Geometry check sheet. Reference: the model listing, model coordinates, mm. Give positions to 0.01 mm unless a question says otherwise; leave off trailing zeros. Write each loop counter-clockwise with the first axis right and the second up, starting at its lowest first coordinate (ties: lowest second). Pieces come first, ordered by that corner, then holes. Notation, with made-up numbers: M 34,-6.5 L 72,-6.5 A25 ccw 72,9.5 Z; hole C 58.25,39.25 d5. An arc over 180 degrees is marked long. Write each question's results on one line, items separated by ' | '.
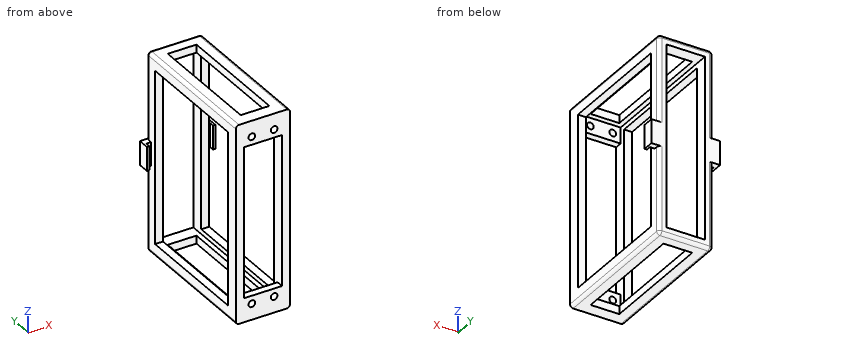
Autodesk Inventor part; units mm, degrees
ref_plane "YZ Plane" through (0, 0, 0) normal (1, 0, 0) x (0, 1, 0)
ref_plane "XZ Plane" through (0, 0, 0) normal (0, 1, 0) x (-1, 0, 0)
ref_plane "XY Plane" through (0, 0, 0) normal (0, 0, 1) x (1, 0, 0)
sketch "Sketch1" plane through (0, 0, 0) normal (0, 1, 0) x (-1, 0, 0)
  point P0 (0, 0)
sketch "Sketch2" plane through (0, 0, 0) normal (0, 1, 0) x (-1, 0, 0)
  line L0 (34.7144, 60.4703) -> (0.7144, 60.4703)
  line L1 (0.7144, 60.4703) -> (0.7144, -63.8297)
  line L2 (0.7144, -63.8297) -> (34.7144, -63.8297)
  line L3 (34.7144, -63.8297) -> (34.7144, 60.4703)
  point P0 (0, 0)
  dimension "d0" = 124.3
  dimension "d1" = 34
extrude "Extrusion1" add sketch "Sketch2" along normal blind 90
sketch "Sketch3" plane through (0, 90, 0) normal (0, 1, 0) x (1, 0, 0)
  line L0 (-34.7144, -60.4703) -> (-0.7144, -60.4703) construction
  line L1 (-0.7144, -60.4703) -> (-0.7144, 63.8297) construction
  line L2 (-0.7144, 63.8297) -> (-34.7144, 63.8297) construction
  line L3 (-34.7144, 63.8297) -> (-34.7144, -60.4703) construction
  line L4 (-29.7144, 58.8297) -> (-5.7144, 58.8297)
  line L5 (-5.7144, 58.8297) -> (-5.7144, -55.4703)
  line L6 (-5.7144, -55.4703) -> (-29.7144, -55.4703)
  line L7 (-29.7144, -55.4703) -> (-29.7144, 58.8297)
  point P0 (0, 0)
  dimension "d4" = 114.3
  dimension "d5" = 24
  dimension "d6" = 5
  dimension "d7" = 5
  dimension "d8" = 5
  dimension "d9" = 5
extrude "Extrusion2" cut sketch "Sketch3" against normal blind 85.5
sketch "Sketch4" plane through (-0.7144, 0, 60.4703) normal (1, 0, 0) x (0, 0, -1)
  line L0 (124.3, 0) -> (124.3, 90) construction
  line L1 (0, 90) -> (124.3, 90) construction
  line L2 (54.65, 90) -> (69.65, 90)
  line L3 (69.65, 90) -> (69.65, 83)
  line L4 (69.65, 83) -> (54.65, 83)
  line L5 (54.65, 83) -> (54.65, 90)
  point P0 (60.4703, 0)
  dimension "d12" = 15
  dimension "d13" = 7
  dimension "d14" = 0
  dimension "d15" = 54.65
extrude "Extrusion3" add sketch "Sketch4" along normal blind 4.5
sketch "Sketch5" plane through (-34.7144, 0, -63.8297) normal (-1, 0, 0) x (0, 0, 1)
  line L0 (124.3, 0) -> (124.3, 90) construction
  line L1 (0, 90) -> (124.3, 90) construction
  line L2 (54.65, 90) -> (69.65, 90)
  line L3 (69.65, 90) -> (69.65, 83)
  line L4 (69.65, 83) -> (54.65, 83)
  line L5 (54.65, 83) -> (54.65, 90)
  point P0 (63.8297, 0)
  dimension "d18" = 7
  dimension "d19" = 15
  dimension "d20" = 0
  dimension "d21" = 54.65
extrude "Extrusion4" add sketch "Sketch5" along normal blind 4.5
sketch "Sketch6" plane through (-34.7144, 83, -9.1797) normal (0, -1, 0) x (1, 0, 0)
  line L0 (0, 15) -> (0, 0) construction
  line L1 (0, 15) -> (-4.5, 15) construction
  line L2 (-3, 0) -> (0, 0)
  line L3 (0, 0) -> (0, 15)
  line L4 (0, 15) -> (-3, 15)
  line L5 (-3, 15) -> (-3, 0)
  point P0 (34.7144, 9.1797)
  dimension "d24" = 15
  dimension "d25" = 3
  dimension "d26" = 0
  dimension "d27" = 0
extrude "Extrusion5" cut sketch "Sketch6" against normal blind 3
sketch "Sketch7" plane through (-0.7144, 83, -9.1797) normal (0, -1, 0) x (1, 0, 0)
  line L0 (0, 0) -> (0, 15) construction
  line L1 (0, 15) -> (4.5, 15) construction
  line L2 (0, 15) -> (3, 15)
  line L3 (3, 15) -> (3, 0)
  line L4 (3, 0) -> (0, 0)
  line L5 (0, 0) -> (0, 15)
  point P0 (0.7144, 9.1797)
  dimension "d30" = 15
  dimension "d31" = 3
  dimension "d32" = 0
  dimension "d33" = 0
extrude "Extrusion6" cut sketch "Sketch7" against normal blind 3
sketch "Sketch8" plane through (-34.7144, 0, 60.4703) normal (0, 0, 1) x (1, 0, 0)
  line L0 (0, 0) -> (34, 0) construction
  line L1 (34, 0) -> (34, 90) construction
  line L2 (0, 90) -> (34, 90) construction
  line L3 (0, 0) -> (0, 90) construction
  line L4 (8, 82) -> (26, 82)
  line L5 (26, 82) -> (26, 8)
  line L6 (26, 8) -> (8, 8)
  line L7 (8, 8) -> (8, 82)
  point P0 (34.7144, 0)
  dimension "d38" = 8
  dimension "d39" = 8
  dimension "d84" = 8
  dimension "d85" = 8
extrude "Extrusion7" cut sketch "Sketch8" against normal blind 124.3
sketch "Sketch9" plane through (-0.7144, 0, 60.4703) normal (1, 0, 0) x (0, 0, -1)
  line L0 (0, 0) -> (0, 90) construction
  line L1 (0, 0) -> (124.3, 0) construction
  line L2 (124.3, 0) -> (124.3, 90) construction
  line L3 (69.65, 90) -> (124.3, 90) construction
  line L4 (8, 82) -> (116.3, 82)
  line L5 (116.3, 82) -> (116.3, 8)
  line L6 (116.3, 8) -> (8, 8)
  line L7 (8, 8) -> (8, 82)
  point P0 (60.4703, 0)
  dimension "d46" = 8
  dimension "d48" = 8
  dimension "d82" = 8
  dimension "d83" = 8
extrude "Extrusion8" cut sketch "Sketch9" against normal blind 34
sketch "Sketch11" plane through (0, 0, 0) normal (0, -1, 0) x (1, 0, 0)
  line L0 (-34.7144, 60.4703) -> (-0.7144, 60.4703) construction
  line L1 (-34.7144, -63.8297) -> (-34.7144, 60.4703) construction
  line L2 (-0.7144, -63.8297) -> (-34.7144, -63.8297) construction
  line L3 (-0.7144, 60.4703) -> (-0.7144, -63.8297) construction
  circle A0 centre (-24.7144, -53.8297) radius 2.1
  circle A1 centre (-10.7144, -53.8297) radius 2.1
  circle A2 centre (-24.7144, 50.4703) radius 2.1
  circle A3 centre (-10.7144, 50.4703) radius 2.1
  line L4 (-29.7144, -48.8297) -> (-5.7144, -48.8297)
  line L5 (-5.7144, -48.8297) -> (-5.7144, 45.4703)
  line L6 (-5.7144, 45.4703) -> (-29.7144, 45.4703)
  line L7 (-29.7144, 45.4703) -> (-29.7144, -48.8297)
  point P0 (0, 0)
  dimension "d52" = 4.2
  dimension "d53" = 10
  dimension "d54" = 10
  dimension "d55" = 4.2
  dimension "d56" = 10
  dimension "d57" = 10
  dimension "d58" = 4.2
  dimension "d59" = 10
  dimension "d60" = 10
  dimension "d61" = 4.2
  dimension "d62" = 10
  dimension "d63" = 10
  dimension "d66" = 94.3
  dimension "d67" = 24
  dimension "d68" = 5
  dimension "d69" = 5
  dimension "d70" = 5
  dimension "d71" = 5
extrude "Extrusion9" cut sketch "Sketch11" against normal blind 5 contours A0 | A1 | A2 | A3
sketch "Sketch12" plane through (0, 0, 0) normal (0, -1, 0) x (1, 0, 0)
  circle A0 centre (-24.7144, 50.4703) radius 2.1 construction
  circle A1 centre (-24.7144, -53.8297) radius 2.1 construction
  line L0 (-34.7144, -63.8297) -> (-34.7144, 60.4703) construction
  line L1 (-0.7144, 60.4703) -> (-0.7144, -63.8297) construction
  line L2 (-29.7144, -48.8297) -> (-5.7144, -48.8297)
  line L3 (-5.7144, -48.8297) -> (-5.7144, 45.4703)
  line L4 (-5.7144, 45.4703) -> (-29.7144, 45.4703)
  line L5 (-29.7144, 45.4703) -> (-29.7144, -48.8297)
  point P0 (0, 0)
  dimension "d72" = 94.3
  dimension "d73" = 24
  dimension "d74" = 5
  dimension "d75" = 5
  dimension "d76" = 5
  dimension "d77" = 5
extrude "Extrusion10" cut sketch "Sketch12" against normal blind 5
fillet "Fillet1" radius 2 10 edges at (-34.7144, 90, -36.5047) (-34.7144, 90, 33.1453) (-17.7144, 90, 60.4703) (-0.7144, 90, 33.1453) (-0.7144, 90, -36.5047) (-17.7144, 90, -63.8297) (-34.7144, 45, 60.4703) (-0.7144, 45, 60.4703) (-0.7144, 45, -63.8297) (-34.7144, 45, -63.8297)
equation "\"d38\" = d84"
equation "\"d39\" = d84"
equation "\"d85\" = d84"
equation "\"d48\" = d46"
equation "\"d82\" = d48"
equation "\"d83\" = d46"
equation "\"d52\" = d55"
equation "\"d55\" = d61"
equation "\"d58\" = d61"
properties part number "Battery Case2"
Q1. Section check C-C (y = 31). Enter the section's corners in (x, z), then the cut area to 3 significant figures.
Answer key:
outline: M -34.71,-61.83 A2 ccw -32.71,-63.83 L -26.71,-63.83 L -26.71,-58.83 L -29.71,-58.83 L -29.71,-55.83 L -34.71,-55.83 Z; M -34.71,52.47 L -29.71,52.47 L -29.71,55.47 L -26.71,55.47 L -26.71,60.47 L -32.71,60.47 A2 ccw -34.71,58.47 Z; M -8.71,-63.83 L -2.71,-63.83 A2 ccw -0.71,-61.83 L -0.71,-55.83 L -5.71,-55.83 L -5.71,-58.83 L -8.71,-58.83 Z; M -8.71,55.47 L -5.71,55.47 L -5.71,52.47 L -0.71,52.47 L -0.71,58.47 A2 ccw -2.71,60.47 L -8.71,60.47 Z | area: 217 mm2
Q2. Depth check by flat-ended pin: P1, Ø11, axis at x = -17, z = 48.5, coming from the +Y side; P2, Ø5, axis at x = 0.5, y = 87.5, coming from the -Z side; P3, Ø2.5, axis at y = 47.5, z = 58, coming from the +X side. Enter the tip coordinate at first touch or a pass-through.
Answer key:
P1: stops at y = 4.5 | P2: stops at z = -63.7 | P3: stops at x = -0.71
Q3. Section check A-A (z = 3). Enter the section's corners in (x, y).
Answer key:
outline: M -39.21,83 L -37.71,83 L -37.71,86 L -34.71,86 L -34.71,82 L -29.71,82 L -29.71,90 L -39.21,90 Z; M -34.71,0 L -29.71,0 L -29.71,8 L -34.71,8 Z; M -5.71,0 L -0.71,0 L -0.71,8 L -5.71,8 Z; M -5.71,82 L -0.71,82 L -0.71,86 L 2.29,86 L 2.29,83 L 3.79,83 L 3.79,90 L -5.71,90 Z
Q4. Material ranges on probe 1 along X at (y, z) = (6, -37.5); probe 2 along Z at (x, y) = (-27, 39.5); probe 3 along Z at (x, y) = (-4, 55.5), recorded low to high. Write a range as [from, to].
Answer key:
probe 1: x = [-34.71, -29.71], [-5.71, -0.71] | probe 2: z = [-63.83, -58.83], [55.47, 60.47] | probe 3: z = [-63.83, -55.83], [52.47, 60.47]
Q5. Section check B-B (x = -19.5). Enter the section's corners in (y, z), then the cut area to 3 significant figures.
Answer key:
outline: M 0,-63.83 L 8,-63.83 L 8,-58.83 L 4.5,-58.83 L 4.5,-48.83 L 0,-48.83 Z; M 0,45.47 L 4.5,45.47 L 4.5,55.47 L 8,55.47 L 8,60.47 L 0,60.47 Z; M 82,-63.83 L 88,-63.83 A2 ccw 90,-61.83 L 90,-58.83 L 82,-58.83 Z; M 82,55.47 L 90,55.47 L 90,58.47 A2 ccw 88,60.47 L 82,60.47 Z | area: 248 mm2
Q6. Section check D-D (x = -7). Enter the section's corners in (y, z), then the cut area to 3 significant figures.
Answer key:
outline: M 0,-63.83 L 88,-63.83 A2 ccw 90,-61.83 L 90,-58.83 L 4.5,-58.83 L 4.5,-48.83 L 0,-48.83 Z; M 0,45.47 L 4.5,45.47 L 4.5,55.47 L 90,55.47 L 90,58.47 A2 ccw 88,60.47 L 0,60.47 Z | area: 988 mm2
